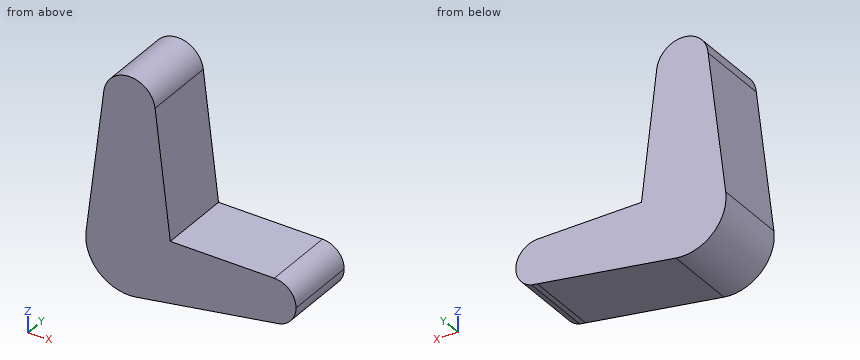
```python
from build123d import *

# Parameters (mm, degrees)
F1_DEPTH = 25


with BuildPart() as f1:
    # F0 (on Front) → F1 (new body)
    with BuildSketch(Plane.XZ):
        with BuildLine():
            Line((13.74659, 7.85846), (8.625084, 50.304803))
            ThreePointArc((8.625084, 50.304803), (-0.198572, 57.949485), (-8.663633, 49.909534))
            Line((-8.663633, 49.909534), (-14.584756, 1.794839))
            ThreePointArc((-14.584756, 1.794839), (-10.238037, -10.541307), (2.219706, -14.526164))
            Line((2.219706, -14.526164), (48.765101, -7.413681))
            ThreePointArc((48.765101, -7.413681), (41.209057, -0.023461), (48.718184, 7.414425))
            Line((48.718184, 7.414425), (13.74659, 7.85846))
        make_face()
        with BuildLine():
            ThreePointArc((56.039065, 0), (53.900434, 5.209822), (48.718184, 7.414425))
            ThreePointArc((48.718184, 7.414425), (41.209057, -0.023461), (48.765101, -7.413681))
            Line((48.765101, -7.413681), (50.703455, -7.117486))
            ThreePointArc((50.703455, -7.117486), (54.557062, -4.447677), (56.039065, 0))
        make_face()
    extrude(amount=F1_DEPTH)


solid = f1.part
```
The listing builds one solid part. Answer for the finished solid, in the listing's coordinates (mm). Give positions to 0.01 mm unless a question says otherwise; leave off trailing zeros. Order: outer loops, then holes, each group sorted by start corner. A loop starts at its lowest first (then second) coordinate and runs counter-clockwise, first axis right, second up.
1) Find section A-A on y = -7.75. Write down the section's boundary in (x, z).
Reported:
outline: (-14.58, 1.79) arc R14.69 ccw to (2.22, -14.53) - (50.7, -7.12) arc R7.42 ccw to (56.04, 0) arc R7.42 ccw to (48.72, 7.41) - (13.75, 7.86) - (8.63, 50.3) arc R8.69 ccw to (-8.66, 49.91) - close
2) Find section C-C on x = 12. Write down the section's boundary in (y, z), then the cut area to 3 significant figures.
Reported:
outline: (-25, -13.03) - (0, -13.03) - (0, 22.33) - (-25, 22.33) - close
area: 884 mm2
3) Consider line 1 along X through (y, z) = (-4.25, 28); line 2 along X through (y, z) = (-12.25, 36); line 3 along Z through (x, y) = (28, -13.75). Determine where each line is inside the solid, lowest interval first.
Reported:
line 1: x = -11.36 to 11.32
line 2: x = -10.38 to 10.35
line 3: z = -10.59 to 7.68
4) Find section B-B on z = -8.5. Write down the section's boundary in (x, y), then the cut area to 3 significant figures.
Reported:
outline: (-11.99, -25) - (41.66, -25) - (41.66, 0) - (-11.99, 0) - close
area: 1,340 mm2
5) Given P1, Ø5, axis at y = -18, z = 20.5, coming from the -X side; P2, Ø6, axis at x = 27, y = -3.5, coming from the +Z side; P3, Ø10, axis at y = -6, z = 25.5, coming from the -X side, each flat-ended and moving along its own axis, determine where each tip first touches the part or whether it passes through.
Reported:
P1: stops at x = -12.59
P2: stops at z = 7.73
P3: stops at x = -12.28
